Verification items for this drawing (mm, ordinates from the low corner). Coordinates: 2 decimals unless noted, no trailing zeros. Order: outer loops, then holes, each group sorted by start corner. A loop starts at its lowest first (then second) coordinate and runs counter-clockwise, first axis right, second up. Notation, with made-up numbers: (35.5, 22.25) -> (77.5, 22.25) arc R25 cw to (77.5, 61.25) -> close; hole circle Ø2 at (74.5, -35.75). An arc over 180 degrees is marked (long way). Write each question's results on one line, items separated by ' | '. Start each with the question number.
(1) Cross-section at A-A on z = 65. Enter the section's corners in (x, y) (1 decimal), and give its area (3 significant figures).
(2) Cross-section at C-C on y = 1.95. Give the number of separate pieces and of enclosed holes in the cut face, and give its area (3 significant figures).
(3) Go/stop test with flat-tipped pins: pin 1 (3 mm diameter, centred on x = 23, y = 4, fed in from +Z); pin 2 (1.5 mm diameter, centred on y = 1.5, z = 34, fed in from -X); pin 3 (2 mm diameter, centred on y = 3.5, z = 82.5, fed in from +X). Record where each tip stops, or that it passes through.
(4) Thickness scan on probe 1 along Z at (x, y) = (7.5, 3.8) (1 decimal); probe 2 along X at (y, z) = (2.15, 19) (1 decimal); probe 3 along Z at (x, y) = (5.5, 4.4) (1 decimal). Record the ranges inside material, lowest first. Write a range as [from, to].
(5) Cross-section at B-B on x = 88.5. Enter the section's corners in (y, z) (1 decimal).
(6) Cross-section at D-D on x = 8. Enter the section's corners in (y, z).
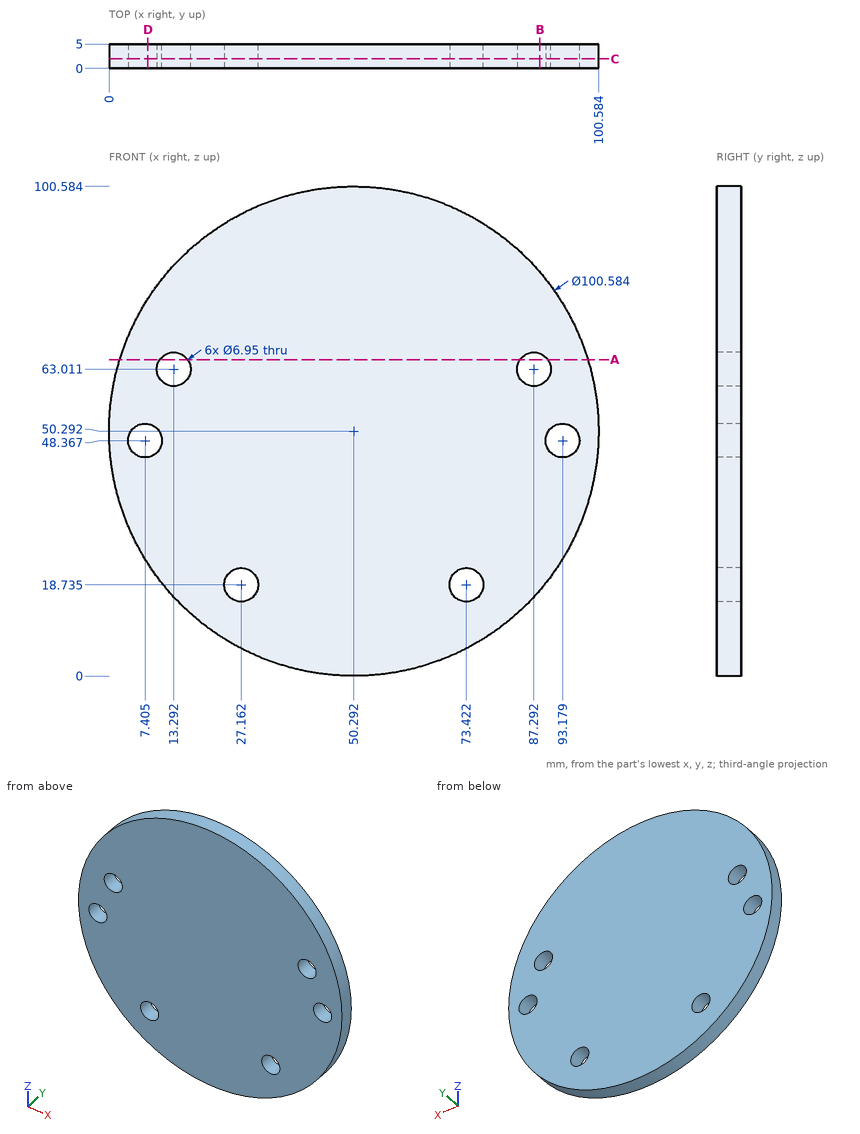
Results are:
1) outline: (2.2, 0) -> (10.4, 0) -> (10.4, 5) -> (2.2, 5) -> close; (16.1, 0) -> (84.4, 0) -> (84.4, 5) -> (16.1, 5) -> close; (90.1, 0) -> (98.4, 0) -> (98.4, 5) -> (90.1, 5) -> close | area: 424 mm2
2) separate pieces: 1 | enclosed holes: 6 | area: 7,720 mm2
3) pin 1: stops at z = 93.47 | pin 2: stops at x = 2.46 | pin 3: stops at x = 89.73
4) probe 1: z = [23.9, 44.9], [51.8, 76.7] | probe 2: x = [10.9, 23.7], [30.6, 70], [76.9, 89.7] | probe 3: z = [27.4, 45.5], [51.3, 73.2]
5) outline: (0, 17.6) -> (5, 17.6) -> (5, 59.8) -> (0, 59.8) -> close; (0, 66.3) -> (5, 66.3) -> (5, 83) -> (0, 83) -> close
6) outline: (0, 23.08) -> (5, 23.08) -> (5, 44.94) -> (0, 44.94) -> close; (0, 51.79) -> (5, 51.79) -> (5, 77.51) -> (0, 77.51) -> close
